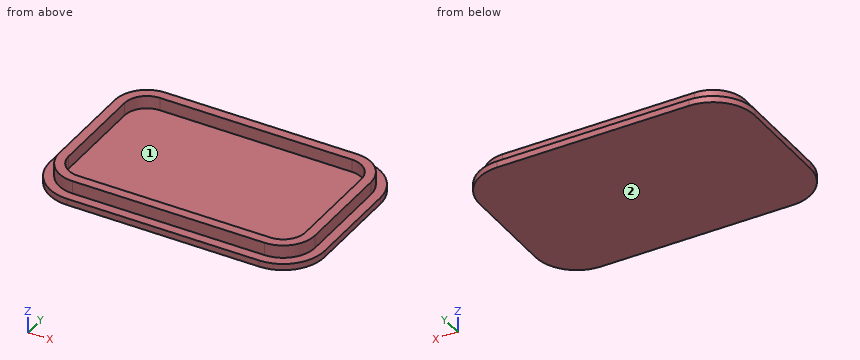
from build123d import *

# Parameters (mm, degrees)
PAD_DEPTH    = 2
PAD001_DEPTH = 6
POCKET_DEPTH = 5


with BuildPart() as part:
    # Sketch001 → Pad (new body)
    with BuildSketch(Plane.XY):
        with BuildLine():
            Line((-43, 15), (-43, -15))
            ThreePointArc((-43, -15), (-39.192388, -24.192388), (-30, -28))
            Line((-30, -28), (30, -28))
            ThreePointArc((30, -28), (39.192388, -24.192388), (43, -15))
            Line((43, -15), (43, 15))
            ThreePointArc((43, 15), (39.192388, 24.192388), (30, 28))
            Line((30, 28), (-30, 28))
            ThreePointArc((-30, 28), (-39.192388, 24.192388), (-43, 15))
        make_face()
    extrude(amount=PAD_DEPTH)

    # Sketch004 → Pad001 (join)
    with BuildSketch(Plane.XY):
        with BuildLine():
            Line((-40, 15), (-40, -15))
            ThreePointArc((-40, -15), (-37.071068, -22.071068), (-30, -25))
            Line((-30, -25), (30, -25))
            ThreePointArc((30, -25), (37.071068, -22.071068), (40, -15))
            Line((40, -15), (40, 15))
            ThreePointArc((40, 15), (37.071068, 22.071068), (30, 25))
            Line((30, 25), (-30, 25))
            ThreePointArc((-30, 25), (-37.071068, 22.071068), (-40, 15))
        make_face()
    extrude(amount=PAD001_DEPTH)

    # Sketch005 → Pocket (cut)
    with BuildSketch(Plane.XY.offset(2)):
        with BuildLine():
            Line((-37, 15), (-37, -15))
            ThreePointArc((-37, -15), (-34.949747, -19.949747), (-30, -22))
            Line((-30, -22), (30, -22))
            ThreePointArc((30, -22), (34.949747, -19.949747), (37, -15))
            Line((37, -15), (37, 15))
            ThreePointArc((37, 15), (34.949747, 19.949747), (30, 22))
            Line((30, 22), (-30, 22))
            ThreePointArc((-30, 22), (-34.949747, 19.949747), (-37, 15))
        make_face()
    extrude(amount=POCKET_DEPTH, mode=Mode.SUBTRACT)


solid = part.part
Build history of the part. All positions in model axes, mm. Face numbers are marked on the shaded views. Coordinates: 2 decimals unless noted, no trailing zeros. Write each loop counter-clockwise with the first axis right and the second up, starting at its lowest first coordinate (ties: lowest second). Pieces come first, ordered by that corner, then holes.
(1) Cut at C-C on y = -2.5. List the corners of the cut face in (x, z), and give its area (3 significant figures).
(2) Cut at B-B on x = -28.5. List the corners of the cut face in (y, z), and give its area (3 significant figures).
(3) Pin check, flat tips, straight feed: pin 1 Ø1.5 at (x, z) = (25.5, 3) entering from +Y; pin 2 Ø2 at (y, z) = (-1, 5) entering from +X; pin 3 Ø2 at (x, z) = (-2.5, 4.5) entering from -Y. Stop position of each tip, or through.
(4) Drill centre lines: line 1 (X direction, y = 4, z = 2.55); line 2 (Y direction, x = -11.5, z = 5.3); line 3 (Z direction, x = -22, y = -21). Where is each one in solid material? Low to high.
(5) Mould opens along Y. For the marked faces 1 and 2 say: pulls with the +Y half, pulls with the -Y half, needs draft (parallel to the pull), parting line crosses it, or undercut.
(6) Cut at A-A on z = 3.75. List the corners of the cut face in (x, y), and give its area (3 significant figures).
Working result:
1. outline: (-43, 0) - (43, 0) - (43, 2) - (40, 2) - (40, 6) - (37, 6) - (37, 2) - (-37, 2) - (-37, 6) - (-40, 6) - (-40, 2) - (-43, 2) - close
1. area: 196 mm2
2. outline: (-28, 0) - (28, 0) - (28, 2) - (25, 2) - (25, 6) - (22, 6) - (22, 2) - (-22, 2) - (-22, 6) - (-25, 6) - (-25, 2) - (-28, 2) - close
2. area: 136 mm2
3. pin 1: stops at y = 25
3. pin 2: stops at x = 40
3. pin 3: stops at y = -25
4. line 1: x = -40 to -37, 37 to 40
4. line 2: y = -25 to -22, 22 to 25
4. line 3: z = 0 to 2
5. face 1: undercut
5. face 2: needs draft
6. outline: (-40, -15) arc R10 ccw to (-30, -25) - (30, -25) arc R10 ccw to (40, -15) - (40, 15) arc R10 ccw to (30, 25) - (-30, 25) arc R10 ccw to (-40, 15) - close; hole (-37, -15) arc R7 ccw to (-30, -22) - (30, -22) arc R7 ccw to (37, -15) - (37, 15) arc R7 ccw to (30, 22) - (-30, 22) arc R7 ccw to (-37, 15) - close
6. area: 700 mm2
